```python
from build123d import *

# Parameters (mm, degrees)
SKETCH1_R           = 1.6
BOSS_EXTRUDE1_DEPTH = 10


with BuildPart() as part:
    # Sketch1 → Boss-Extrude1 (new body)
    with BuildSketch(Plane(origin=(0, 0, 0), x_dir=(1, 0, 0), z_dir=(0, 1, 0))):
        with BuildLine():
            Line((-3, 14.5), (3, 14.5))
            add(Edge.make_bspline(
                [(3, 14.5), (7.114682306, 14.5), (16.320193537, 10.316763311), (31.07742048, 9.595600445), (41.442510879, 11.590070739), (45.709603601, 14.653822942)],
                knots=[0, 0, 0, 0, 0.28514411, 0.663251595, 1, 1, 1, 1], degree=3))
            ThreePointArc((45.709603601, 14.653822942), (65.5, 4.5), (45.709603601, -5.653822942))
            add(Edge.make_bspline(
                [(3, -5.5), (7.114682306, -5.5), (16.320193537, -1.316763311), (31.07742048, -0.595600445), (41.442510879, -2.590070739), (45.709603601, -5.653822942)],
                knots=[0, 0, 0, 0, 0.28514411, 0.663251595, 1, 1, 1, 1], degree=3))
            Line((3, -5.5), (-3, -5.5))
            Line((-3, -5.5), (-3, 14.5))
        make_face()
        with Locations(Location((0, 0, 0), (0, 0, 270))):
            Circle(SKETCH1_R, mode=Mode.SUBTRACT)
        with Locations(Location((0, 9, 0), (0, 0, 270))):
            Circle(SKETCH1_R, mode=Mode.SUBTRACT)
    extrude(amount=BOSS_EXTRUDE1_DEPTH)


solid = part.part
```
Can you work these out from the model? Positions are in its coordinate system, mm. A direction names the side the tool comes from. Coordinates: 2 decimals unless noted, no trailing zeros. Write each loop counter-clockwise with the first axis right and the second up, starting at its lowest first coordinate (ties: lowest second). Pieces come first, ordered by that corner, then holes. Notation, with made-up numbers: M 81.5,-26.5 L 95.5,-26.5 A20 cw 95.5,12.5 Z; hole C -29.75,29 d3. An arc over 180 degrees is marked long. Answer as CSV lines item,"result".
Item 1: Imagine slicing it at D-D on x = 61. List the corners of the cut face in (y, z) for me, plus the area to 3 significant figures.
Geometry results:
outline,"M 0,-14.1 L 10,-14.1 L 10,5.1 L 0,5.1 Z"
area,"192 mm2"
Item 2: I'm going to push flat-ended pins straight in: P1, Ø1, axis at y = 9, z = 0.5, coming from the +X side; P2, Ø1.5, axis at x = 5.5, y = 8, coming from the -Z side; P3, Ø1.8, axis at x = 0, y = 6.5, coming from the -Z side; P4, Ø2.5, axis at x = 0, z = 0, coming from the -Y side. Where does each tip first touch, or does it pass through?
Geometry results:
P1,"stops at x = 64.66"
P2,"stops at z = -14.4"
P3,"stops at z = -14.5"
P4,"passes through"
Item 3: Please list where these lines run through material, in increasing order: line 1 along Z through (x, y) = (26.5, 4.5); line 2 along X through (y, z) = (5.75, -5); line 3 along X through (y, z) = (3.25, -9).
Geometry results:
line 1,"z = -10.09 to 1.09"
line 2,"x = -3 to 65.49"
line 3,"x = -3 to -1.6, 1.6 to 64.66"
Item 4: Imagine slicing it at C-C on y = 1.5. State how many separate pieces and enclosed holes the cut face has, plus the area to 3 significant figures.
Geometry results:
separate pieces,"1"
enclosed holes,"2"
area,"1,130 mm2"
Item 5: Imagine slicing it at B-B on z = -0.5. List the corners of the cut face in (x, y) for me.
Geometry results:
outline,"M -3,0 L -1.52,0 L -1.52,10 L -3,10 Z; M 1.52,0 L 64.84,0 L 64.84,10 L 1.52,10 Z"
Item 6: On a 3-axis mill with a long thin cutter (end or side, diameter ignored), from which of +Z, -Z, +X, -X, +Y, -Y can I reach the whole of each face in a straight line? I mean faces 1 (the cylindrical face through (0.07, 4.93, -10.6)), 2 (the flat face through (0, 5, 5.5)). Say none if no direction works.
Geometry results:
face 1,"+Y, -Y"
face 2,"+Z, -X, +Y, -Y"
Item 7: We'd pull the mould along X, two halves only. Please class faces 3 (the flat face through (-3, 5, -4)), 4 (the cylindrical face through (-0.97, 4.93, -1.27)), 5 (the flat face through (0, 5, -14.5)): +X half, -X half, draft (parallel to the pull), parting line (faces both ways), or undercut.
Geometry results:
face 3,"-X half"
face 4,"undercut"
face 5,"draft"
Item 8: Imagine slicing it at A-A on x = 0. List the corners of the cut face in (y, z) for me, plus the area to 3 significant figures.
Geometry results:
outline,"M 0,-14.5 L 10,-14.5 L 10,-10.6 L 0,-10.6 Z; M 0,-7.4 L 10,-7.4 L 10,-1.6 L 0,-1.6 Z; M 0,1.6 L 10,1.6 L 10,5.5 L 0,5.5 Z"
area,"136 mm2"
